Autodesk Inventor part; units mm, degrees
ref_plane "YZ Plane" through (0, 0, 0) normal (1, 0, 0) x (0, 1, 0)
ref_plane "XZ Plane" through (0, 0, 0) normal (0, 1, 0) x (-1, 0, 0)
ref_plane "XY Plane" through (0, 0, 0) normal (0, 0, 1) x (1, 0, 0)
sketch "Sketch1" plane through (0, 0, 0) normal (0, 1, 0) x (-1, 0, 0)
  circle A0 centre (0, 0) radius 7.5
  line L0 (1.5, 1.5) -> (-1.5, -1.5) construction
  line L1 (-1.5, 1.5) -> (1.5, -1.5) construction
  arc A1 (7.5, 0) -> (12.5, 0) centre (10, 4.3301) ccw
  line L2 (0, 0) -> (5.3033, -5.3033)
  line L3 (0, 0) -> (6.9291, -2.8701)
  line L4 (0, 0) -> (7.5, 0) construction
  line L5 (0, 0) -> (7.3559, -1.4632)
  line L6 (0, 0) -> (7.5, 0) construction
  line L7 (0, 0) -> (7.4639, -0.7351)
  line L8 (0, 0) -> (7.5, 0) construction
  line L9 (12.5, 0) -> (12.5, -0.7351)
  arc A2 (7.4639, -0.7351) -> (7.5, 0) centre (0, 0) ccw
  arc A3 (7.3559, -1.4632) -> (12.5, -0.7351) centre (9.3293, 3.1309) ccw
  arc A4 (6.4952, 3.75) -> (10.8253, 6.25) centre (6.4952, 8.75) ccw
  line L10 (10.8253, 6.25) -> (11.1929, 5.6134)
  arc A5 (7.102, 2.4108) -> (11.1929, 5.6134) centre (6.5139, 7.3761) ccw
  arc A6 (3.75, 6.4952) -> (6.25, 10.8253) centre (1.25, 10.8253) ccw
  line L11 (6.25, 10.8253) -> (6.8866, 10.4578)
  arc A7 (4.9451, 5.6388) -> (6.8866, 10.4578) centre (1.9532, 9.6448) ccw
  arc A8 (0, 7.5) -> (0, 12.5) centre (-4.3301, 10) ccw
  line L12 (0, 12.5) -> (0.7351, 12.5)
  arc A9 (1.4632, 7.3559) -> (0.7351, 12.5) centre (-3.1309, 9.3293) ccw
  arc A10 (-3.75, 6.4952) -> (-6.25, 10.8253) centre (-8.75, 6.4952) ccw
  line L13 (-6.25, 10.8253) -> (-5.6134, 11.1929)
  arc A11 (-2.4108, 7.102) -> (-5.6134, 11.1929) centre (-7.3761, 6.5139) ccw
  arc A12 (-6.4952, 3.75) -> (-10.8253, 6.25) centre (-10.8253, 1.25) ccw
  line L14 (-10.8253, 6.25) -> (-10.4578, 6.8866)
  arc A13 (-5.6388, 4.9451) -> (-10.4578, 6.8866) centre (-9.6448, 1.9532) ccw
  arc A14 (-7.5, 0) -> (-12.5, 0) centre (-10, -4.3301) ccw
  line L15 (-12.5, 0) -> (-12.5, 0.7351)
  arc A15 (-7.3559, 1.4632) -> (-12.5, 0.7351) centre (-9.3293, -3.1309) ccw
  arc A16 (-6.4952, -3.75) -> (-10.8253, -6.25) centre (-6.4952, -8.75) ccw
  line L16 (-10.8253, -6.25) -> (-11.1929, -5.6134)
  arc A17 (-7.102, -2.4108) -> (-11.1929, -5.6134) centre (-6.5139, -7.3761) ccw
  arc A18 (-3.75, -6.4952) -> (-6.25, -10.8253) centre (-1.25, -10.8253) ccw
  line L17 (-6.25, -10.8253) -> (-6.8866, -10.4578)
  arc A19 (-4.9451, -5.6388) -> (-6.8866, -10.4578) centre (-1.9532, -9.6448) ccw
  arc A20 (0, -7.5) -> (0, -12.5) centre (4.3301, -10) ccw
  line L18 (0, -12.5) -> (-0.7351, -12.5)
  arc A21 (-1.4632, -7.3559) -> (-0.7351, -12.5) centre (3.1309, -9.3293) ccw
  arc A22 (3.75, -6.4952) -> (6.25, -10.8253) centre (8.75, -6.4952) ccw
  line L19 (6.25, -10.8253) -> (5.6134, -11.1929)
  arc A23 (2.4108, -7.102) -> (5.6134, -11.1929) centre (7.3761, -6.5139) ccw
  arc A24 (6.4952, -3.75) -> (10.8253, -6.25) centre (10.8253, -1.25) ccw
  line L20 (10.8253, -6.25) -> (10.4578, -6.8866)
  arc A25 (5.6388, -4.9451) -> (10.4578, -6.8866) centre (9.6448, -1.9532) ccw
  line L21 (1.85, -1.85) -> (-1.85, -1.85)
  line L22 (-1.85, -1.85) -> (-1.85, 1.85)
  line L23 (-1.85, 1.85) -> (1.85, 1.85)
  line L24 (1.85, 1.85) -> (1.85, -1.85)
  line L25 (1.85, -1.85) -> (-1.85, 1.85) construction
  line L26 (-1.85, -1.85) -> (1.85, 1.85) construction
  point P0 (7.102, 2.4108)
  point P1 (6.4952, 3.75)
  point P2 (4.9451, 5.6388)
  point P3 (3.75, 6.4952)
  point P4 (1.4632, 7.3559)
  point P5 (0, 7.5)
  point P6 (-2.4108, 7.102)
  point P7 (-3.75, 6.4952)
  point P8 (-5.6388, 4.9451)
  point P9 (-6.4952, 3.75)
  point P10 (-7.3559, 1.4632)
  point P11 (-7.5, 0)
  point P12 (-1.4632, -7.3559)
  point P13 (0, -7.5)
  point P14 (2.4108, -7.102)
  point P15 (3.75, -6.4952)
  dimension "d0" = 15
  dimension "d1" = 3
  dimension "d2" = 3
  dimension "d3" = 5
  dimension "d4" = 5
  dimension "d5" = 22.5
  dimension "d6" = 11.25
  dimension "d7" = 5.625
  dimension "d13" = 5
  dimension "d16" = 360
  dimension "d20" = 3.7
  dimension "d21" = 3.7
extrude "Extrusion1" add sketch "Sketch1" along normal blind 50 contours A0 L7 L24 L23 L22 L21 L2 | A1 L9 A3 A0 | A0 A4 L10 A5 | A0 L5 L24 L7 | A0 L3 L24 L5 | A0 A6 L11 A7 | A0 L2 L24 L3 | A24 L20 A25 A0 | A0 A8 L12 A9 | A22 L19 A23 A0 | A0 A10 L13 A11 | A20 L18 A21 A0 | A0 A12 L14 A13 | A18 L17 A19 A0 | A0 A14 L15 A15 | A16 L16 A17 A0
sketch "Sketch2" plane through (12.5, 0, 0) normal (1, 0, 0) x (0, 0, -1)
  point P0 (0, 0)
sketch "Sketch3" plane through (0, 50, 0) normal (0, 1, 0) x (1, 0, 0)
  point P0 (0, 0)
sketch "Sketch4" plane through (-6.25, 0, 10.8253) normal (-0.5, 0, 0.866) x (0.866, 0, 0.5)
  point P0 (0, 0)
sketch "Sketch5" plane through (0, 50, 0) normal (0, 1, 0) x (1, 0, 0)
  point P0 (0, 0)
equation "\"BendRadius\" = Thickness"
equation "\"BendReliefWidth\" = Thickness"
equation "\"BendReliefDepth\" = 0.5 * Thickness"
equation "\"CornerReliefSize\" = 4 * Thickness"
equation "\"MinimumRemnant\" = 2 * Thickness"
equation "\"TransitionRadius\" = BendRadius"
equation "\"JacobiRadiusSize\" = BendRadius"
equation "\"GapSize\" = Thickness"
Here's how the part is built. I have some questions about the finished solid (model axes, mm). A direction names the side the tool comes from. Give positions to 0.01 mm unless a question says otherwise; leave off trailing zeros. Order: outer loops, then holes, each group sorted by start corner. A loop starts at its lowest first (then second) coordinate and runs counter-clockwise, first axis right, second up. Notation, with made-up numbers: (84.5, 38.25) -> (103.5, 38.25) arc R28 ccw to (103.5, 75.25) -> close; hole circle Ø9 at (5, -4.5). An arc over 180 degrees is marked (long way). Use CSV: the item, a comma, the result in double quotes. Start each with the question number.
Item 1: Suppose I cut it at C-C (x = 4.25). List the corners of the cut face in (y, z) for me.
Item 2: On a 3-axis mill with a long thin cutter (end or side, diameter ignored), from which of +Z, -Z, +X, -X, +Y, -Y can I reach the whole of each face in a straight line? I mean faces 3 (the cylindrical face through (-8.36, 24.65, -5.6)), 4 (the cylindrical face through (10.04, 24.65, 0.67)). Say none if no direction works.
Item 3: Suppose I cut it at B-B (z = -8). List the corners of the cut face in (x, y) for me.
Item 4: If I drill on probe 1 along Z at (x, y) = (10, 22); probe 2 along X at (y, z) = (36.5, -8.5); probe 3 along X at (y, z) = (12.5, 5.5), over which ranges is the centre line in solid material (lowest first)? Write a range as [from, to].
Item 5: Suppose I cut it at A-A (x = 8). List the corners of the cut face in (y, z) for me, and give its area (3 significant figures).
Item 6: I'm going to push flat-ended pins straight in: P1, Ø1.5, axis at x = 4, y = 25.5, coming from the +Z side; P2, Ø1.5, axis at x = -3, y = 27.5, coming from the +Z side. Where does each tip first touch, or does it pass through?
Item 7: Thinking about a two-plate mould opening in Z: for faces 1 (the flat face through (2, 0, -2)), 2 (the cylindrical face through (0.67, 24.65, -10.04)), which applies, pulls with the +Z half, pulls with the -Z half, needs draft (parallel to the pull), parting line crosses it, or undercut?
Item 8: Suppose I cut it at D-D (x = -3.25). List the corners of the cut face in (y, z) for me.
Answer block:
1,outline,"(0, -6.83) -> (50, -6.83) -> (50, 6.18) -> (0, 6.18) -> close; (0, 8.67) -> (50, 8.67) -> (50, 10.42) -> (0, 10.42) -> close"
2,face 3,"-X, +Y, -Y"
2,face 4,"+Y, -Y"
3,outline,"(-3.98, 0) -> (-2.6, 0) -> (-2.6, 50) -> (-3.98, 50) -> close; (0.25, 0) -> (1.69, 0) -> (1.69, 50) -> (0.25, 50) -> close; (5.38, 0) -> (6.67, 0) -> (6.67, 50) -> (5.38, 50) -> close"
4,probe 1,"z = [-5.18, -3.79], [0.67, 1.82], [6.18, 6.94]"
4,probe 2,"x = [-4.17, -2.79], [0.44, 1.8], [5.68, 6.82]"
4,probe 3,"x = [-11.15, -10.29], [-5.1, 5.1], [6.12, 8.19]"
5,outline,"(0, -3.98) -> (50, -3.98) -> (50, -2.6) -> (0, -2.6) -> close; (0, 0.25) -> (50, 0.25) -> (50, 1.69) -> (0, 1.69) -> close; (0, 5.38) -> (50, 5.38) -> (50, 6.67) -> (0, 6.67) -> close"
5,area,"206 mm^2"
6,P1,"stops at z = 10.77"
6,P2,"stops at z = 7.15"
7,face 1,"needs draft"
7,face 2,"undercut"
8,outline,"(0, -9.34) -> (50, -9.34) -> (50, 6.76) -> (0, 6.76) -> close"
